from build123d import *

# Parameters (mm, degrees)
SKETCH_1_W          = 25
SKETCH_1_H          = 10
EXTRUDE_1_DEPTH     = 85
SKETCH_2_R          = 6
CUT_EXTRUDE_1_DEPTH = 90.162772501
M3X0_5_1_D          = 2.5
M3X0_5_1_DEPTH      = 11.5
M3X0_5_1_TIP        = 0.751075774


with BuildPart() as part:
    # ｽｹｯﾁ1 → ﾎﾞｽ - 押し出し1 (new body)
    with BuildSketch(Plane(origin=(0, 0, 0), x_dir=(1, 0, 0), z_dir=(0, 1, 0))):
        with Locations((12.5, 5)):
            Rectangle(SKETCH_1_W, SKETCH_1_H)
    extrude(amount=EXTRUDE_1_DEPTH)

    # ｽｹｯﾁ2 → ｶｯﾄ - 押し出し1 (cut, through all)
    with BuildSketch(Plane.XY):
        with Locations((12.5, 70)):
            Circle(SKETCH_2_R)
    extrude(amount=-CUT_EXTRUDE_1_DEPTH, mode=Mode.SUBTRACT)

    # M3x0.5 ねじ穴1
    with Locations(Plane.XZ):
        with Locations((20, -5), (5, -5)):
            Hole(M3X0_5_1_D / 2, depth=M3X0_5_1_DEPTH)
            with Locations((0, 0, -(M3X0_5_1_DEPTH + M3X0_5_1_TIP / 2))):  # 118° drill point
                Cone(0, M3X0_5_1_D / 2, M3X0_5_1_TIP, mode=Mode.SUBTRACT)


solid = part.part
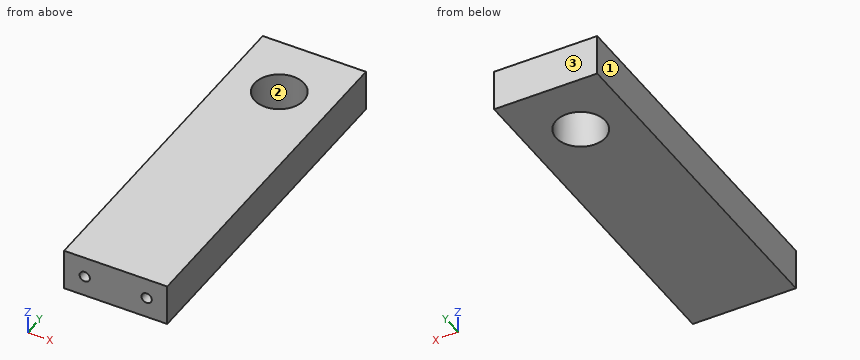
Here's how the part is built. I have some questions about the finished solid (model axes, mm). Face numbers are marked on the shaded views. Coordinates: 2 decimals unless noted, no trailing zeros. Loops run counter-clockwise (first coordinate to the right, second up) from the corner with the lowest first, then second, coordinate; pieces in that order, holes last.
1. Imagine slicing it at C-C, the plane z = -2.25. Please give me the cut outline in (x, y).
2. If we mould it in two halves opening along X, with no side actions, what happens to the marked faces 1, 2 and 3? For each: pulls with the +X half, pulls with the -X half, needs draft (parallel to the pull), parting line crosses it, or undercut.
3. I need wall thicknesses on L1, parallel to X at y = 4.75, z = -5; L2, parallel to X at y = 8.5, z = -5.5; L3, parallel to Z at x = 5, y = 3.25. Which ranges of each line are inside material? Lowest first, please.
4. Imagine slicing it at A-A, the plane x = 12.5. Please give me the cut outline in (y, z).
5. Imagine slicing it at B-B, the plane y = 70. Please give me the cut outline in (x, z), and give its area (3 significant figures).
6. For P1, Ø9.5, axis at x = 12.5, y = 70, coming from the -Z side, with a flat end and sliding along its axis, tell me the tip position at first contact or that it passes through.
Taken from the geometry:
1. outline: (0, 0) - (25, 0) - (25, 85) - (0, 85) - close; hole circle Ø12 at (12.5, 70)
2. face 1: pulls with the -X half
2. face 2: undercut
2. face 3: needs draft
3. L1: x = 0 to 3.75, 6.25 to 18.75, 21.25 to 25
3. L2: x = 0 to 3.85, 6.15 to 18.85, 21.15 to 25
3. L3: z = -10 to -6.25, -3.75 to 0
4. outline: (0, -10) - (64, -10) - (64, 0) - (0, 0) - close; (76, -10) - (85, -10) - (85, 0) - (76, 0) - close
5. outline: (0, -10) - (6.5, -10) - (6.5, 0) - (0, 0) - close; (18.5, -10) - (25, -10) - (25, 0) - (18.5, 0) - close
5. area: 130 mm2
6. P1: passes through
